Check sheet for the modelled part. Datum: model origin and axes. Units: mm. Round coordinates to 2 decimals unless told otherwise and drop trailing zeros. Loops run counter-clockwise (first coordinate to the right, second up) from the corner with the lowest first, then second, coordinate; pieces in that order, holes last. Notation, with made-up numbers: (33.25, -25.75) - (92.25, -25.75) arc R29 ccw to (92.25, 5.25) - close; hole circle Ø11 at (-32.5, -16.5). An arc over 180 degrees is marked (long way). Put each result on its own line as item: value.
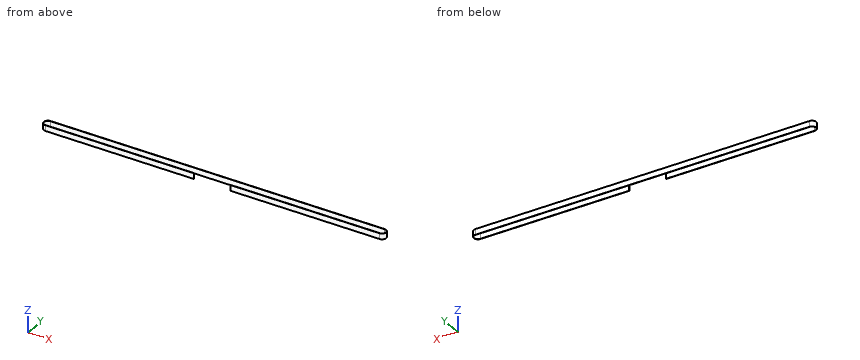
```python
from build123d import *

# Parameters (mm, degrees)
SKETCH2_W               = 8.5
SKETCH2_H               = 0.5
CUT_EXTRUDE1_DEPTH      = 262.181067078
CUT_EXTRUDE1_DEPTH_BACK = 262.181067078
SKETCH3_W               = 56
SKETCH3_H               = 40


with BuildPart() as part:
    # Sweep1: sweep along a path in Sketch1
    with BuildLine(Plane.XY) as sweep1_path:
        Line((-254.75, 5.82), (254.75, 5.82))
        ThreePointArc((254.75, 5.82), (260.57, 0), (254.75, -5.82))
        Line((254.75, -5.82), (-254.75, -5.82))
        ThreePointArc((-254.75, -5.82), (-260.57, 0), (-254.75, 5.82))
    # Sketch2 → Sweep1 (sweep)
    with BuildSketch(Plane(origin=(0, 0, 0), x_dir=(0, 0, -1), z_dir=(1, 0, 0))):
        with Locations((0, 6.07)):
            Rectangle(SKETCH2_W, SKETCH2_H)
    sweep(path=sweep1_path.line)

    # Sketch3 → Cut-Extrude1 (cut, two sides: drawn at the far end of the back side and taken through both)
    with BuildSketch(Plane.XY.offset(-CUT_EXTRUDE1_DEPTH_BACK)):
        with Locations((0, -20)):
            Rectangle(SKETCH3_W, SKETCH3_H)
    extrude(amount=CUT_EXTRUDE1_DEPTH + CUT_EXTRUDE1_DEPTH_BACK, mode=Mode.SUBTRACT)


solid = part.part
```
Item 1: Thickness scan on line 1 (Y direction, x = -222, z = 1); line 2 (X direction, y = 0.5, z = 1.75); line 3 (X direction, y = -0.25, z = 0.5). Record the ranges inside material, lowest first. Write a range as from..to.
Filled sheet:
line 1: -6.32..-5.82, 5.82..6.32
line 2: -261.05..-260.55, 260.55..261.05
line 3: -261.07..-260.56, 260.56..261.07
Item 2: Section check C-C on z = -0.25. Enter the section's corners in (x, y).
Filled sheet:
outline: (-254.75, -6.32) - (-28, -6.32) - (-28, -5.82) - (-254.75, -5.82) arc R5.82 cw to (-254.75, 5.82) - (254.75, 5.82) arc R5.82 cw to (254.75, -5.82) - (28, -5.82) - (28, -6.32) - (254.75, -6.32) arc R6.32 ccw to (254.75, 6.32) - (-254.75, 6.32) arc R6.32 ccw to start
Item 3: Section check A-A on x = -201. Enter the section's corners in (y, z).
Filled sheet:
outline: (-6.32, -4.25) - (-5.82, -4.25) - (-5.82, 4.25) - (-6.32, 4.25) - close; (5.82, -4.25) - (6.32, -4.25) - (6.32, 4.25) - (5.82, 4.25) - close
Item 4: Section check B-B on y = 0. Enter the section's corners in (x, z).
Filled sheet:
outline: (-261.07, -4.25) - (-260.57, -4.25) - (-260.57, 4.25) - (-261.07, 4.25) - close; (260.57, -4.25) - (261.07, -4.25) - (261.07, 4.25) - (260.57, 4.25) - close
Item 5: Go/stop test with a flat-tipped pin: pin 1 (0.6 mm diameter, centred on y = -6, z = -0.5, fed in from -X). Record where the tip stops, or that it passes through.
Filled sheet:
pin 1: x = -257.48
